from build123d import *

# Parameters (mm, degrees)
SKETCH1_R           = 13.5
BOSS_EXTRUDE1_DEPTH = 30
SKETCH2_R           = 1.25
CUT_EXTRUDE1_DEPTH  = 4


with BuildPart() as part:
    # Sketch1 → Boss-Extrude1 (new, symmetric)
    with BuildSketch(Plane(origin=(0, 0, 0), x_dir=(0, 0, -1), z_dir=(1, 0, 0))):
        Circle(SKETCH1_R)
    extrude(amount=BOSS_EXTRUDE1_DEPTH, both=True)

    # Sketch2 → Cut-Extrude1 (cut)
    with BuildSketch(Plane.ZY.offset(30)):
        with Locations((0, 10)):
            Circle(SKETCH2_R)
        with Locations((8.660254038, 5)):
            Circle(SKETCH2_R)
        with Locations((8.660254038, -5)):
            Circle(SKETCH2_R)
        with Locations((0, -10)):
            Circle(SKETCH2_R)
        with Locations((-8.660254038, -5)):
            Circle(SKETCH2_R)
        with Locations((-8.660254038, 5)):
            Circle(SKETCH2_R)
    cut_extrude1 = extrude(amount=-CUT_EXTRUDE1_DEPTH, mode=Mode.SUBTRACT)

    # Mirror1: Cut-Extrude1 across plane
    add(cut_extrude1.mirror(Plane(origin=(0, 0, 0), x_dir=(0, 0, 1), z_dir=(1, 0, 0))), mode=Mode.SUBTRACT)


solid = part.part
Read the model definition and answer for the solid it produces. Units are mm, in the model's axes. A direction names the side the tool comes from. Give positions to 0.01 mm unless a question says otherwise; leave off trailing zeros. Write each loop counter-clockwise with the first axis right and the second up, starting at its lowest first coordinate (ties: lowest second). Pieces come first, ordered by that corner, then holes. Notation, with made-up numbers: (26.5, 50.25) -> (39.5, 50.25) arc R28 ccw to (39.5, 81.25) -> close; hole circle Ø5 at (43.5, -7.5). An arc over 180 degrees is marked (long way). Answer as a JSON object with one key per item and string values. Group by question number.
1) Consider L1, parallel to Y at x = -27.25, z = 0; L2, parallel to Y at x = -2.5, z = 0; L3, parallel to Y at x = -17, z = 6.25. Determine where each line is inside the solid, lowest interval first. Write a range as from..to.
2) The mould has two halves that part along Z. Classify faces 3 (the flat face through (30, 0, 0)), 4 (the cylindrical face through (-28.028, -8.946, 0.672)): +Z half, -Z half, draft (parallel to the pull), parting line (faces both ways), or undercut.
3) Find section C-C (x = 14). Write down the section's boundary in (y, z), and give its area (3 significant figures).
4) Find section B-B (y = 5). Write down the section's boundary in (x, z), and give its area (3 significant figures).
5) Find section D-D (y = 10). Write down the section's boundary in (x, z).
6) Find section A-A (z = 0). Write down the section's boundary in (x, y), and give its area (3 significant figures).
7) Each of these flat-tipped pins is pushed along its axis until it touches: P1, Ø2, axis at x = 18.5, z = 4, coming from the +Y side; P2, Ø2, axis at x = 5, z = 8.5, coming from the +Y side (3 decimals); P3, Ø3, axis at x = 16, y = 7.5, coming from the +Z side. Where does it stop, or does it pass through?
8) A tool of negligible diameter and unlimited length cuts with its end or side. For faces 1 (the cylindrical face through (28.03, 11.24, -0.16)), 2 (the cylindrical face through (-28.028, 4.521, -7.506)), from which of +Z, -Z, +X, -X, +Y, -Y can it reach the whole face along a straight path? Write none if from no direction.
Values follow:
{
 "1": {"L1": "y = -13.5..-11.25, -8.75..8.75, 11.25..13.5", "L2": "y = -13.5..13.5", "L3": "y = -11.97..11.97"},
 "2": {"face 3": "draft", "face 4": "undercut"},
 "3": {"outline": "circle Ø27 at (0, 0)", "area": "573 mm2"},
 "4": {"outline": "(-30, -12.54) -> (30, -12.54) -> (30, -9.91) -> (26, -9.91) -> (26, -7.41) -> (30, -7.41) -> (30, 7.41) -> (26, 7.41) -> (26, 9.91) -> (30, 9.91) -> (30, 12.54) -> (-30, 12.54) -> (-30, 9.91) -> (-26, 9.91) -> (-26, 7.41) -> (-30, 7.41) -> (-30, -7.41) -> (-26, -7.41) -> (-26, -9.91) -> (-30, -9.91) -> close", "area": "1,460 mm2"},
 "5": {"outline": "(-30, -9.07) -> (30, -9.07) -> (30, -1.25) -> (26, -1.25) -> (26, 1.25) -> (30, 1.25) -> (30, 9.07) -> (-30, 9.07) -> (-30, 1.25) -> (-26, 1.25) -> (-26, -1.25) -> (-30, -1.25) -> close"},
 "6": {"outline": "(-30, -13.5) -> (30, -13.5) -> (30, -11.25) -> (26, -11.25) -> (26, -8.75) -> (30, -8.75) -> (30, 8.75) -> (26, 8.75) -> (26, 11.25) -> (30, 11.25) -> (30, 13.5) -> (-30, 13.5) -> (-30, 11.25) -> (-26, 11.25) -> (-26, 8.75) -> (-30, 8.75) -> (-30, -8.75) -> (-26, -8.75) -> (-26, -11.25) -> (-30, -11.25) -> close", "area": "1,580 mm2"},
 "7": {"P1": "stops at y = 13.16", "P2": "stops at y = 11.225", "P3": "stops at z = 12.09"},
 "8": {"face 1": "+X", "face 2": "-X"}
}
